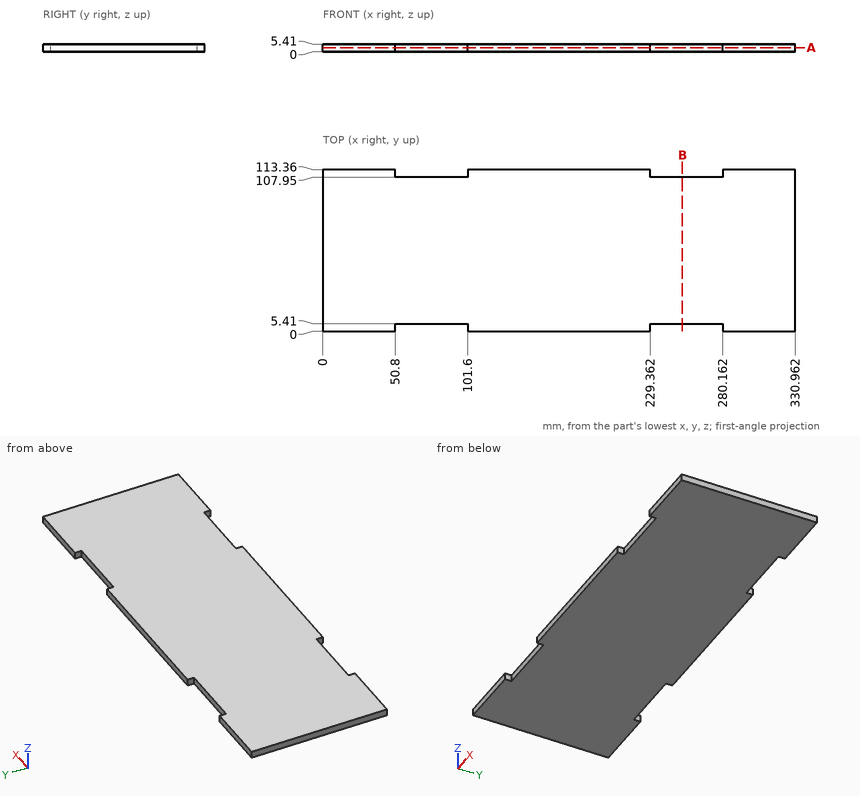
Source: three-view drawing plus pictorial views. Frame: mm from the lowest corner of the part. Coordinates: 2 decimals unless noted, no trailing zeros. Order: outer loops, then holes, each group sorted by start corner. A loop starts at its lowest first (then second) coordinate and runs counter-clockwise, first axis right, second up. Notation, with made-up numbers: M 21.25,4.25 L 29.25,4.25 A26 cw 29.25,34.25 Z; hole C 47,75 d5. An arc over 180 degrees is marked long. One line per question, with ' | ' between items. Start each with the question number.
Item 1: Cut plane A-A, the plane z = 2.95. Return the cut outline in (x, y).
Item 2: Cut plane B-B, the plane x = 252. Return the cut outline in (y, z), then the cut area to 3 significant figures.
Item 3: Pin query (flat end, axial travel): pin 1 Ø2 at (x, z) = (248.5, 5) entering from +Y. Return the tip coordinate at first contact, or that it passes through.
Item 4: Ray query, probe 1 along Y at (x, z) = (246, 0.75). Return the intervals inside material, ascending. Write a range as [from, to].
A:
1) outline: M 0,0 L 50.8,0 L 50.8,5.41 L 101.6,5.41 L 101.6,0 L 229.36,0 L 229.36,5.41 L 280.16,5.41 L 280.16,0 L 330.96,0 L 330.96,113.36 L 280.16,113.36 L 280.16,107.95 L 229.36,107.95 L 229.36,113.36 L 101.6,113.36 L 101.6,107.95 L 50.8,107.95 L 50.8,113.36 L 0,113.36 Z
2) outline: M 5.41,0 L 107.95,0 L 107.95,5.41 L 5.41,5.41 Z | area: 555 mm2
3) pin 1: stops at y = 107.95
4) probe 1: y = [5.41, 107.95]
